Source: CAD feature listing. Evaluate the final solid. Frame: model axes, mm. Face numbers are marked on the shaded views. A direction names the side the tool comes from. Round coordinates to 2 decimals unless told otherwise and drop trailing zeros. Loops run counter-clockwise (first coordinate to the right, second up) from the corner with the lowest first, then second, coordinate; pieces in that order, holes last. Notation, with made-up numbers: M -34,-11 L 9,-11 A32 cw 9,28 Z; hole C 45.25,76.5 d4. An arc over 180 degrees is marked long. Answer as a JSON object with one key per item and string values.
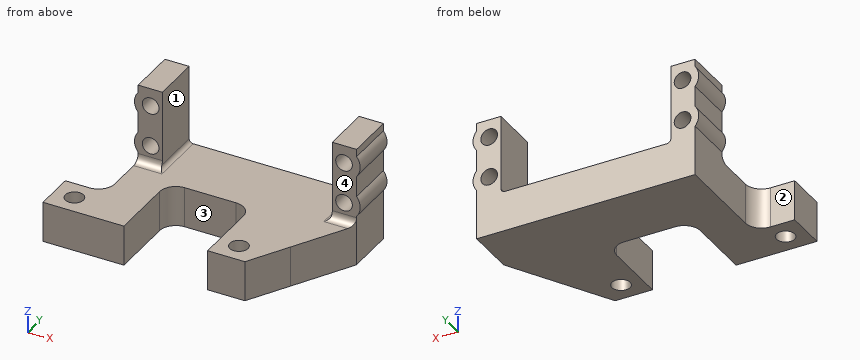
from build123d import *

# Parameters (mm, degrees)
SKETCH1_W            = 54
SKETCH1_H            = 26.5
BOSS_EXTRUDE1_DEPTH  = 10
CUT_EXTRUDE1_DEPTH   = 10
SKETCH3_W            = 15
SKETCH3_H            = 10
SKETCH3_W_2          = 10
BOSS_EXTRUDE2_DEPTH  = 10
CUT_EXTRUDE2_DEPTH   = 10
SKETCH5_W            = 20.679801083
SKETCH5_H            = 5
CUT_EXTRUDE3_DEPTH   = 10
SKETCH6_W            = 6
SKETCH6_H            = 12
BOSS_EXTRUDE3_DEPTH  = 19.5
SKETCH7_R            = 2.06
CUT_EXTRUDE4_DEPTH   = 37.5
SKETCH8_R            = 2.06
BOSS_EXTRUDE4_DEPTH  = 12
FILLET1_R            = 2
FILLET2_R            = 1
FILLET1_OF_MIRROR1_R = 2
FILLET2_OF_MIRROR1_R = 1
SKETCH9_R            = 2.25
CUT_EXTRUDE5_DEPTH   = 10
CUT_EXTRUDE6_DEPTH   = 10
SKETCH11_W           = 20.679801083
SKETCH11_H           = 10
CUT_EXTRUDE7_DEPTH   = 10
FILLET3_R            = 4
SKETCH12_W           = 10
SKETCH12_H           = 10
BOSS_EXTRUDE5_DEPTH  = 10
SKETCH13_R           = 2.25
CUT_EXTRUDE8_DEPTH   = 10
FILLET4_R            = 4


with BuildPart() as part:
    # Sketch1 → Boss-Extrude1 (new body)
    with BuildSketch(Plane.XY):
        Rectangle(SKETCH1_W, SKETCH1_H)
    boss_extrude1 = extrude(amount=BOSS_EXTRUDE1_DEPTH)

    # Sketch2 → Cut-Extrude1 (cut)
    with BuildSketch(Plane(origin=(0, 0, 0), x_dir=(-1, 0, 0), z_dir=(0, 0, -1))):
        Polygon((-27, 1.161007253), (-18.679801083, -13.25), (-27, -13.25), align=None)
    extrude(amount=-CUT_EXTRUDE1_DEPTH, mode=Mode.SUBTRACT)

    # Sketch3 → Boss-Extrude2 (add)
    with BuildSketch(Plane.XZ.offset(13.25)):
        with Locations((11.179801083, 5)):
            Rectangle(SKETCH3_W, SKETCH3_H)
        with Locations((-22, 5)):
            Rectangle(SKETCH3_W_2, SKETCH3_H)
    extrude(amount=BOSS_EXTRUDE2_DEPTH)

    # Sketch4 → Cut-Extrude2 (cut)
    with BuildSketch(Plane(origin=(0, 0, 0), x_dir=(-1, 0, 0), z_dir=(0, 0, -1))):
        Polygon((-18.679801083, -13.25), (-12.906298391, -23.25), (-18.679801083, -23.25), align=None)
    extrude(amount=-CUT_EXTRUDE2_DEPTH, mode=Mode.SUBTRACT)

    # Sketch5 → Cut-Extrude3 (cut)
    with BuildSketch(Plane(origin=(0, 0, 0), x_dir=(-1, 0, 0), z_dir=(0, 0, -1))):
        with Locations((6.660099458, -10.75)):
            Rectangle(SKETCH5_W, SKETCH5_H)
    extrude(amount=-CUT_EXTRUDE3_DEPTH, mode=Mode.SUBTRACT)

    # Sketch6 → Boss-Extrude3 (add)
    with BuildSketch(Plane.XY.offset(10)):
        with Locations((24, 7.25)):
            Rectangle(SKETCH6_W, SKETCH6_H)
    boss_extrude3 = extrude(amount=BOSS_EXTRUDE3_DEPTH)

    # Sketch7 → Cut-Extrude4 (cut, through all)
    with BuildSketch(Plane(origin=(0, 13.25, 0), x_dir=(1, 0, 0), z_dir=(0, 1, 0))):
        with Locations((23.9, -25.1)):
            Circle(SKETCH7_R)
        with Locations((23.9, -14.9)):
            Circle(SKETCH7_R)
    cut_extrude4 = extrude(amount=-CUT_EXTRUDE4_DEPTH, mode=Mode.SUBTRACT)

    # Sketch8 → Boss-Extrude4 (add)
    with BuildSketch(Plane(origin=(0, 13.25, 0), x_dir=(1, 0, 0), z_dir=(0, 1, 0))):
        with BuildLine():
            Line((21, -27.854995463), (21, -22.345004537))
            ThreePointArc((21, -22.345004537), (27.9, -25.1), (21, -27.854995463))
        make_face()
        with Locations((23.9, -25.1)):
            Circle(SKETCH8_R, mode=Mode.SUBTRACT)
        with BuildLine():
            Line((21, -17.654995463), (21, -12.145004537))
            ThreePointArc((21, -12.145004537), (27.9, -14.9), (21, -17.654995463))
        make_face()
        with Locations((23.9, -14.9)):
            Circle(SKETCH8_R, mode=Mode.SUBTRACT)
    boss_extrude4 = extrude(amount=-BOSS_EXTRUDE4_DEPTH)

    # Fillet1
    fillet1_edges = [part.edges().sort_by_distance(p)[0] for p in [
        (24, 1.25, 10),
    ]]
    fillet(fillet1_edges, radius=FILLET1_R)

    # Fillet2
    fillet2_edges = [part.edges().sort_by_distance(p)[0] for p in [
        (21, 7.25, 10),
    ]]
    fillet(fillet2_edges, radius=FILLET2_R)

    # Mirror1: Boss-Extrude1, Boss-Extrude3, Cut-Extrude4, Boss-Extrude4 across plane
    add(boss_extrude1.mirror(Plane(origin=(0, 0, 0), x_dir=(0, 0, 1), z_dir=(1, 0, 0))))
    add(boss_extrude3.mirror(Plane(origin=(0, 0, 0), x_dir=(0, 0, 1), z_dir=(1, 0, 0))))
    add(cut_extrude4.mirror(Plane(origin=(0, 0, 0), x_dir=(0, 0, 1), z_dir=(1, 0, 0))), mode=Mode.SUBTRACT)
    add(boss_extrude4.mirror(Plane(origin=(0, 0, 0), x_dir=(0, 0, 1), z_dir=(1, 0, 0))))

    # Fillet1 of Mirror1
    fillet1_of_mirror1_edges = [part.edges().sort_by_distance(p)[0] for p in [
        (-24, 1.25, 10),
    ]]
    fillet(fillet1_of_mirror1_edges, radius=FILLET1_OF_MIRROR1_R)

    # Fillet2 of Mirror1
    fillet2_of_mirror1_edges = [part.edges().sort_by_distance(p)[0] for p in [
        (-21, 7.25, 10),
    ]]
    fillet(fillet2_of_mirror1_edges, radius=FILLET2_OF_MIRROR1_R)

    # Sketch9 → Cut-Extrude5 (cut)
    with BuildSketch(Plane.XY.offset(10)):
        with Locations((8.679801083, -18.25)):
            Circle(SKETCH9_R)
    extrude(amount=-CUT_EXTRUDE5_DEPTH, mode=Mode.SUBTRACT)

    # Sketch10 → Cut-Extrude6 (cut)
    with BuildSketch(Plane(origin=(0, 0, 0), x_dir=(-1, 0, 0), z_dir=(0, 0, -1))):
        Polygon((-27, 1.161007253), (-18.679801083, -13.25), (-27, -13.25), align=None)
    extrude(amount=-CUT_EXTRUDE6_DEPTH, mode=Mode.SUBTRACT)

    # Sketch11 → Cut-Extrude7 (cut)
    with BuildSketch(Plane(origin=(0, 0, 0), x_dir=(-1, 0, 0), z_dir=(0, 0, -1))):
        with Locations((6.660099458, -8.25)):
            Rectangle(SKETCH11_W, SKETCH11_H)
    extrude(amount=-CUT_EXTRUDE7_DEPTH, mode=Mode.SUBTRACT)

    # Fillet3
    fillet3_edges = [part.edges().sort_by_distance(p)[0] for p in [
        (-17, -3.25, 5),
        (3.679801083, -3.25, 5),
    ]]
    fillet(fillet3_edges, radius=FILLET3_R)

    # Sketch12 → Boss-Extrude5 (add)
    with BuildSketch(Plane.XY.offset(10)):
        with Locations((-32, -18.25)):
            Rectangle(SKETCH12_W, SKETCH12_H)
    extrude(amount=-BOSS_EXTRUDE5_DEPTH)

    # Sketch13 → Cut-Extrude8 (cut)
    with BuildSketch(Plane.XY.offset(10)):
        with Locations((-32, -18.25)):
            Circle(SKETCH13_R)
    extrude(amount=-CUT_EXTRUDE8_DEPTH, mode=Mode.SUBTRACT)

    # Fillet4
    fillet4_edges = [part.edges().sort_by_distance(p)[0] for p in [
        (-27, -13.25, 5),
    ]]
    fillet(fillet4_edges, radius=FILLET4_R)


solid = part.part
Item 1: Section A-A on x = -23.9. Return the cut outline in (y, z), then the cut area to 3 significant figures.
Answer sheet:
{"outline": "M -23.25,0 L 13.25,0 L 13.25,12.84 L 1.25,12.84 L 1.25,12 A2 cw -0.75,10 L -23.25,10 Z; M 1.25,16.96 L 13.25,16.96 L 13.25,23.04 L 1.25,23.04 Z; M 1.25,27.16 L 13.25,27.16 L 13.25,29.5 L 1.25,29.5 Z", "area": "501 mm²"}
Item 2: Section D-D on y = 5.5. Return the cut outline in (x, z).
Answer sheet:
{"outline": "M -27,0 L 27,0 L 27,12.37 A4 ccw 27,17.43 L 27,22.57 A4 ccw 27,27.63 L 27,29.5 L 21,29.5 L 21,11 A1 cw 20,10 L -20,10 A1 cw -21,11 L -21,29.5 L -27,29.5 L -27,27.63 A4 ccw -27,22.57 L -27,17.43 A4 ccw -27,12.37 Z; hole C -23.9,14.9 d4.12; hole C -23.9,25.1 d4.12; hole C 23.9,14.9 d4.12; hole C 23.9,25.1 d4.12"}
Item 3: Line query: probe 1 along Z at (x, y) = (-23.9, 5.75); probe 2 along X at (y, z) = (-18, 8.25); probe 3 along Y at (x, z) = (-32, 2.5). Output: solid intervals per line, ascending. Write a range as from..to.
Answer sheet:
{"probe 1": "z = 0..12.84, 16.96..23.04, 27.16..29.5", "probe 2": "x = -37..-34.24, -29.76..-17, 3.68..6.44, 10.92..15.94", "probe 3": "y = -23.25..-20.5, -16..-13.25"}
Item 4: Section C-C on z = 7.25. Return the cut outline in (x, y).
Answer sheet:
{"outline": "M -37,-23.25 L -17,-23.25 L -17,-7.25 A4 cw -13,-3.25 L -0.32,-3.25 A4 cw 3.68,-7.25 L 3.68,-23.25 L 12.91,-23.25 L 27,1.16 L 27,13.25 L -27,13.25 L -27,-9.25 A4 cw -31,-13.25 L -37,-13.25 Z; hole C -32,-18.25 d4.5; hole C 8.68,-18.25 d4.5"}
Item 5: Access query for the marked faces 1, 2, 3 and 4. Directions: +Z, -Z, +X, -X, +Y, -Y. A direction counts if a zero-diameter tool reaches every point of the face in a straight line with its end or side. Return the directions, or none.
Answer sheet:
{"face 1": "+Z, +Y, -Y", "face 2": "+Z, -Z, -X, +Y", "face 3": "+Z, -Z, -Y", "face 4": "+Z, +X, -X, -Y"}
Item 6: Section B-B on z = 19.5. Return the cut outline in (x, y), then the cut area to 3 significant figures.
Answer sheet:
{"outline": "M -27,1.25 L -21,1.25 L -21,13.25 L -27,13.25 Z; M 21,1.25 L 27,1.25 L 27,13.25 L 21,13.25 Z", "area": "144 mm²"}
Item 7: Contact query for flat-ended pins moving along their axis: pin 1 Ø8 at (y, z) = (-14, 15.5) entering from -X; pin 2 Ø5 at (x, y) = (18.5, -0.5) entering from +Z; pin 3 Ø10 at (x, z) = (17, 16) entering from -Y; pin 4 Ø9.5 at (y, z) = (10, 7) entering from +X. Output: stop coordinate, or through.
Answer sheet:
{"pin 1": "passes through", "pin 2": "stops at z = 10.41", "pin 3": "stops at y = 1.25", "pin 4": "stops at x = 27"}
